Verification items for this drawing (mm, ordinates from the low corner). Coordinates: 2 decimals unless noted, no trailing zeros. Order: outer loops, then holes, each group sorted by start corner. A loop starts at its lowest first (then second) coordinate and runs counter-clockwise, first axis right, second up. Notation, with made-up numbers: (11, -25) -> (51, -25) arc R6 ccw to (51, -16) -> close; hole circle Ø3 at (9, 35). An arc over 180 degrees is marked (long way). Write each question's results on one line, items separated by ' | '. Start each with the question number.
(1) Cross-section at C-C on x = 59. Enter the section's corners in (y, z).
(2) Draft check along Y on the marked faces 1, 2 and 3. Enter one of: +Y half, -Y half, draft (parallel to the pull), parting line (faces both ways), or undercut.
(3) Thickness scan on probe 1 along Y at (x, z) = (50.5, 6) (1 decimal); probe 2 along Z at (x, y) = (40.5, 18.5); probe 3 along Z at (x, y) = (61.5, 89). Record the ranges inside material, lowest first. Write a range as [from, to].
(4) Cross-section at B-B on y = 65. Enter the section's corners in (x, z) (1 decimal), and give its area (3 significant figures).
(5) Go/stop test with flat-tipped pins: pin 1 (2 mm diameter, centred on y = 17, z = 17, fed in from -X) (1 decimal); pin 2 (4.5 mm diameter, centred on x = 23, z = 18, fed in from -Y); pin 3 (5 mm diameter, centred on x = 22.225, y = 47.625, fed in from +Z). Record where each tip stops, or that it passes through.
(6) Cross-section at A-A on x = 32. Enter the section's corners in (y, z) (1 decimal), and give its area (3 significant figures).
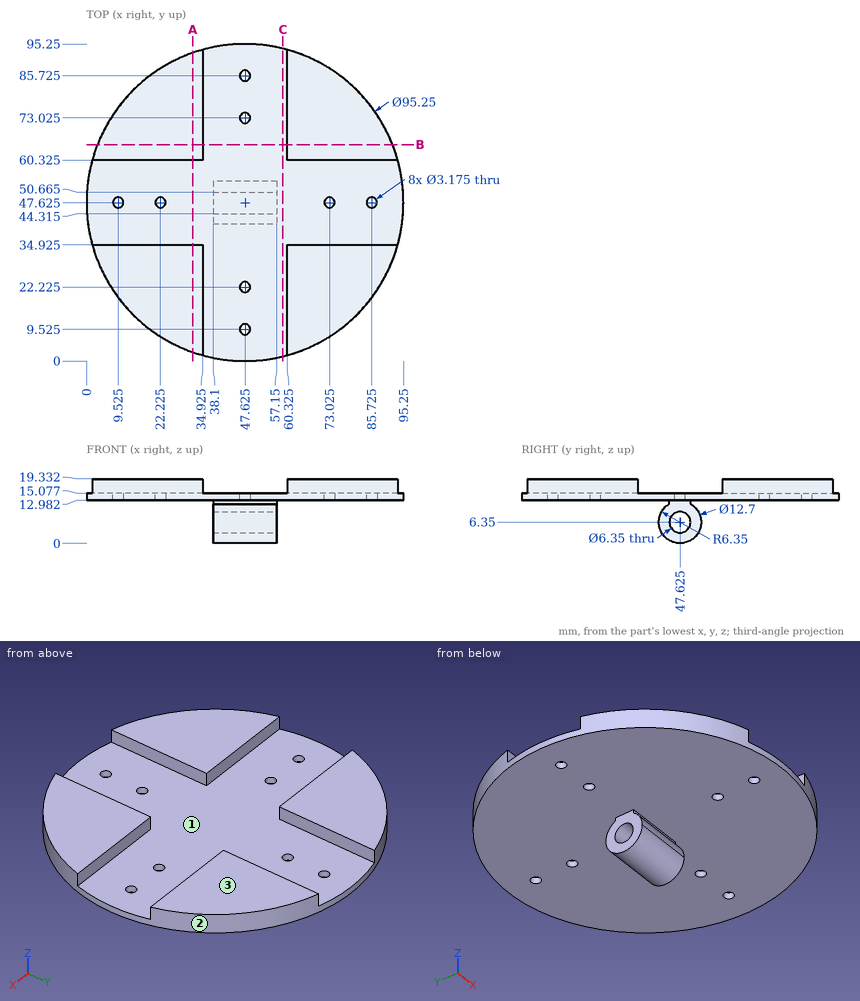
Results are:
1) outline: (1.38, 12.98) -> (93.87, 12.98) -> (93.87, 15.08) -> (1.38, 15.08) -> close
2) face 1: undercut | face 2: parting line | face 3: draft
3) probe 1: y = [41.3, 44.5], [50.8, 54] | probe 2: z = [12.98, 15.08] | probe 3: z = [12.98, 19.33]
4) outline: (3.3, 13) -> (92, 13) -> (92, 19.3) -> (60.3, 19.3) -> (60.3, 15.1) -> (34.9, 15.1) -> (34.9, 19.3) -> (3.3, 19.3) -> close | area: 455 mm2
5) pin 1: stops at x = 10.3 | pin 2: stops at y = 5.58 | pin 3: stops at z = 15.08
6) outline: (2.6, 13) -> (92.6, 13) -> (92.6, 19.3) -> (60.3, 19.3) -> (60.3, 15.1) -> (34.9, 15.1) -> (34.9, 19.3) -> (2.6, 19.3) -> close | area: 463 mm2
